from build123d import *

# Parameters (mm, degrees)
SKETCH1_W      = 42.667
SKETCH1_H      = 32
EXTRUDE1_DEPTH = 0.3
SKETCH2_W      = 34.544
SKETCH2_H      = 25.908
EXTRUDE2_DEPTH = 1
SHELL1_T       = 0.5


with BuildPart() as part:
    # Sketch1 → Extrude1 (new body)
    with BuildSketch(Plane(origin=(0, 0, 0), x_dir=(1, 0, 0), z_dir=(0, 1, 0))):
        with Locations((21.3335, -16)):
            Rectangle(SKETCH1_W, SKETCH1_H)
    extrude(amount=EXTRUDE1_DEPTH)

    # Sketch2 → Extrude2 (add)
    with BuildSketch(Plane(origin=(0, 0.3, 0), x_dir=(-1, 0, 0), z_dir=(0, 1, 0))):
        with Locations((-21.3335, 16)):
            Rectangle(SKETCH2_W, SKETCH2_H)
    extrude(amount=EXTRUDE2_DEPTH)

    # Shell1
    shell1_openings = [part.faces().sort_by_distance(p)[0] for p in [
        (21.3335, 0, 16),
    ]]
    offset(amount=SHELL1_T, openings=shell1_openings, kind=Kind.INTERSECTION)


solid = part.part
Check sheet for the modelled part. Datum: model origin and axes. Units: mm. A direction names the side the tool comes from. Give positions to 0.01 mm unless a question says otherwise; leave off trailing zeros. Loops run counter-clockwise (first coordinate to the right, second up) from the corner with the lowest first, then second, coordinate; pieces in that order, holes last. Notation, with made-up numbers: M 60.5,63 L 100.5,63 A20 ccw 100.5,89 Z; hole C 5.5,69.25 d10. An arc over 180 degrees is marked long. Use a Markdown table: item, result. Add a question column.
Q1. Go/stop test with a flat-tipped pin: pin 1 (1 mm diameter, centred on x = 38, z = 15, fed in from -Y). Record where the tip stops, or that it passes through.
Q2. Sectioned sample at B-B, the plane z = 11.5. Record the cut outline in (x, y), then the cut area to 3 significant figures.
Q3. Scan lines: line 1 along Z through (x, y) = (40, 0.1); line 2 along X through (y, z) = (1, 7); line 3 along Z through (x, y) = (12, 1.2). Record each from-to range of solid material in increasing order. Write a range as [from, to].
Q4. Sectioned sample at C-C, the plane x = 3. Record the cut outline in (y, z), then the cut area to 3 significant figures.
Q5. Tool access check on faces 1 (the flat face through (22, 1, 28.954)), 2 (the flat face through (39.106, 1, 16)), 3 (the flat face through (22, 1, 29.454)), 4 (the flat face through (3.562, 1, 16)). Record the directions out of +Z, -Z, +X, -X, +Y, -Y that give a thin tool (end or side, any length) a straight path to the whole face; none if there is none.
Q6. Sectioned sample at A-A, the plane x = 10.5. Record the cut outline in (y, z).
Q7. Mould release check, pull along Z, two halves, no side actions. Record for faces 5 (the flat face through (22, 1, 2.546)), 6 (the flat face through (22, 1.8, 16)), 7 (the flat face through (38.606, 1, 16)): pulls with the +Z half, pulls with the -Z half, needs draft (parallel to the pull), parting line crosses it, or undercut.
Verdict:
| question | item | result |
|---|---|---|
| 1 | pin 1 | y = 1.3 |
| 2 | outline | M -0.5,0 L 0,0 L 0,0.3 L 4.06,0.3 L 4.06,1.3 L 38.61,1.3 L 38.61,0.3 L 42.67,0.3 L 42.67,0 L 43.17,0 L 43.17,0.8 L 39.11,0.8 L 39.11,1.8 L 3.56,1.8 L 3.56,0.8 L -0.5,0.8 Z |
| 2 | area | 23.1 mm^2 |
| 3 | line 1 | [-0.5, 0], [32, 32.5] |
| 3 | line 2 | [3.56, 4.06], [38.61, 39.11] |
| 3 | line 3 | [2.55, 3.05], [28.95, 29.45] |
| 4 | outline | M 0,-0.5 L 0.8,-0.5 L 0.8,32.5 L 0,32.5 L 0,32 L 0.3,32 L 0.3,0 L 0,0 Z |
| 4 | area | 16.8 mm^2 |
| 5 | face 1 | -Y |
| 5 | face 2 | +Z, -Z, +X, +Y |
| 5 | face 3 | +Z, +X, -X, +Y |
| 5 | face 4 | +Z, -Z, -X, +Y |
| 6 | outline | M 0,-0.5 L 0.8,-0.5 L 0.8,2.55 L 1.8,2.55 L 1.8,29.45 L 0.8,29.45 L 0.8,32.5 L 0,32.5 L 0,32 L 0.3,32 L 0.3,28.95 L 1.3,28.95 L 1.3,3.05 L 0.3,3.05 L 0.3,0 L 0,0 Z |
| 7 | face 5 | pulls with the -Z half |
| 7 | face 6 | needs draft |
| 7 | face 7 | undercut |
